Build history of the part. All positions in model axes, mm. A direction names the side the tool comes from. Give positions to 0.01 mm unless a question says otherwise; leave off trailing zeros. Order: outer loops, then holes, each group sorted by start corner. A loop starts at its lowest first (then second) coordinate and runs counter-clockwise, first axis right, second up. Notation, with made-up numbers: (89.5, 35.25) -> (95.5, 35.25) arc R26 cw to (95.5, 68.25) -> close; hole circle Ø5 at (55, 26.25). An arc over 180 degrees is marked (long way). Use a Markdown table: item, result. Add a question column.
```python
from build123d import *

# Parameters (mm, degrees)
SKETCH1_R           = 1.1
BOSS_EXTRUDE1_DEPTH = 5
SKETCH2_W           = 16
SKETCH2_H           = 12
BOSS_EXTRUDE2_DEPTH = 15
CUT_EXTRUDE1_START  = -5.5
SKETCH3_W           = 9
SKETCH3_H           = 14
CUT_EXTRUDE1_DEPTH  = 9.5
SKETCH4_R           = 1
CUT_EXTRUDE2_DEPTH  = 16
FILLET2_R           = 0.5
SKETCH5_R           = 1.9
CUT_EXTRUDE3_DEPTH  = 1
FILLET3_R           = 1
CUT_EXTRUDE4_START  = -0.5
SKETCH6_R           = 2
CUT_EXTRUDE4_DEPTH  = 5.5
FILLET4_R           = 0.5


with BuildPart() as part:
    # Sketch1 → Boss-Extrude1 (new body)
    with BuildSketch(Plane.XY):
        with BuildLine():
            ThreePointArc((0, 4.5), (-4.5, 0), (0, -4.5))
            Line((0, -4.5), (50, -4.5))
            Line((50, -4.5), (50, 4.5))
            Line((50, 4.5), (0, 4.5))
        make_face()
        Circle(SKETCH1_R, mode=Mode.SUBTRACT)
    extrude(amount=BOSS_EXTRUDE1_DEPTH)

    # Sketch2 → Boss-Extrude2 (add)
    with BuildSketch(Plane(origin=(0, 4.5, 0), x_dir=(1, 0, 0), z_dir=(0, 1, 0))):
        with Locations((58, 1)):
            Rectangle(SKETCH2_W, SKETCH2_H)
    extrude(amount=-BOSS_EXTRUDE2_DEPTH)

    # Sketch3 → Cut-Extrude1 (cut)
    with BuildSketch(Plane(origin=(0, 4.5, 0), x_dir=(1, 0, 0), z_dir=(0, 1, 0)).offset(CUT_EXTRUDE1_START)):
        with Locations((57.5, 2)):
            Rectangle(SKETCH3_W, SKETCH3_H)
    extrude(amount=-CUT_EXTRUDE1_DEPTH, mode=Mode.SUBTRACT)

    # Sketch4 → Cut-Extrude2 (cut)
    with BuildSketch(Plane(origin=(66, 0, 0), x_dir=(0, 0, -1), z_dir=(1, 0, 0))):
        with Locations((1, -6.5)):
            Circle(SKETCH4_R)
    extrude(amount=-CUT_EXTRUDE2_DEPTH, mode=Mode.SUBTRACT)

    # Fillet2
    fillet2_edges = [part.edges().sort_by_distance(p)[0] for p in [
        (53, -6.5, 0),
    ]]
    fillet(fillet2_edges, radius=FILLET2_R)

    # Sketch5 → Cut-Extrude3 (cut)
    with BuildSketch(Plane(origin=(66, 0, 0), x_dir=(0, 0, -1), z_dir=(1, 0, 0))):
        with Locations((1, -6.5)):
            Circle(SKETCH5_R)
    extrude(amount=-CUT_EXTRUDE3_DEPTH, mode=Mode.SUBTRACT)

    # Fillet3
    fillet3_edges = [part.edges().sort_by_distance(p)[0] for p in [
        (53, -10.5, -1),
        (51.5, -10.5, 5),
        (53, -5.75, 5),
        (53, -5.75, -7),
        (51.5, -10.5, -7),
        (64, -10.5, 5),
        (62, -5.75, -7),
        (62, -5.75, 5),
        (64, -10.5, -7),
        (62, -10.5, -1),
    ]]
    fillet(fillet3_edges, radius=FILLET3_R)

    # Sketch6 → Cut-Extrude4 (cut)
    with BuildSketch(Plane.ZY.offset(-50).offset(CUT_EXTRUDE4_START)):
        with Locations((-1, -6.5)):
            Circle(SKETCH6_R)
    extrude(amount=CUT_EXTRUDE4_DEPTH, mode=Mode.SUBTRACT)

    # Fillet4
    fillet4_edges = [part.edges().sort_by_distance(p)[0] for p in [
        (-1.1, 0, 5),
        (-1.1, 0, 0),
    ]]
    fillet(fillet4_edges, radius=FILLET4_R)


solid = part.part
```
(1) Band-saw the part on B-B on z = -1. Give the cut face in (x, y).
(2) Pin check, flat tips, straight feed: pin 1 Ø4.5 at (y, z) = (-5.5, -1.5) entering from -X; pin 2 Ø2.5 at (y, z) = (-6.5, -1) entering from -X; pin 3 Ø3.5 at (x, y) = (0, 0) entering from -Z; pin 4 Ø3 at (x, y) = (34, -6.5) entering from -Z. Stop position of each tip, or through.
(3) Wall check: probe 1 along X at (y, z) = (-3.5, -5); probe 2 along Y at (x, z) = (51.45, -1); probe 3 along Z at (x, y) = (50.35, -6.5). Give the ranges that are in metal, low to high.
(4) Band-saw the part on A-A on y = -6.5. State how many separate pieces and enclosed holes the cut face has, plus the area to 3 significant figures.
(5) Tool access for faces 1 (the face through (65.507, -4.616, -0.753)), 2 (the face through (62, -5, -1)), 3 (the face through (50.254, -8.452, -1.434)), 4 (the face through (25, -4.5, 2)), 5 (the face through (51, -10.5, -1)): list every direction of +Z, -Z, +X, -X, +Y, -Y with a clear straight run to the whole face (end or side of a thin tool).
(6) Band-saw the part on C-C on y = 0. Give the cut face in (x, z).
(7) Mould opens along Y. For faces 6 (the face through (57, -1, -1)), 7 (the face through (63.52, -5.51, -0.87)), 8 (the face through (22, 0, 0)) say: released by +Y, released by -Y, zero draft, split by the parting line, or undercut.
(8) Band-saw the part on D-D on z = -4. Give the cut face in (x, y), plus the area to 3 significant figures.
Response:
| question | item | result |
|---|---|---|
| 1 | outline | (50, -10.5) -> (52, -10.5) arc R1 ccw to (53, -9.5) -> (53, -8) arc R0.5 ccw to (52.5, -7.5) -> (50.5, -7.5) -> (50.5, -8.5) -> (50, -8.5) -> close; (50, -4.5) -> (50.5, -4.5) -> (50.5, -5.5) -> (52.5, -5.5) arc R0.5 ccw to (53, -5) -> (53, -1) -> (62, -1) -> (62, -5.5) -> (65, -5.5) -> (65, -4.6) -> (66, -4.6) -> (66, 4.5) -> (50, 4.5) -> close; (62, -9.5) arc R1 ccw to (63, -10.5) -> (66, -10.5) -> (66, -8.4) -> (65, -8.4) -> (65, -7.5) -> (62, -7.5) -> close |
| 2 | pin 1 | stops at x = -2.37 |
| 2 | pin 2 | stops at x = 50.5 |
| 2 | pin 3 | stops at z = 0 |
| 2 | pin 4 | passes through |
| 3 | probe 1 | x = 50 to 53, 62 to 66 |
| 3 | probe 2 | y = -10.5 to -7.5, -5.5 to 4.5 |
| 3 | probe 3 | z = -7 to -3, 1 to 5 |
| 4 | separate pieces | 4 |
| 4 | enclosed holes | 0 |
| 4 | area | 66.2 mm² |
| 5 | face 1 | +X |
| 5 | face 2 | +Z, -Z, -Y |
| 5 | face 3 | -X |
| 5 | face 4 | +Z, -Z, -X, -Y |
| 5 | face 5 | +Z, -Z, +X, -X, -Y |
| 6 | outline | (-4.5, 0) -> (-1.6, 0) arc R0.5 ccw to (-1.1, 0.5) -> (-1.1, 4.5) arc R0.5 ccw to (-1.6, 5) -> (-4.5, 5) -> close; (1.1, 0.5) arc R0.5 ccw to (1.6, 0) -> (50, 0) -> (50, -7) -> (66, -7) -> (66, 5) -> (1.6, 5) arc R0.5 ccw to (1.1, 4.5) -> close |
| 7 | face 6 | released by -Y |
| 7 | face 7 | undercut |
| 7 | face 8 | zero draft |
| 8 | outline | (50, -10.5) -> (52, -10.5) arc R1 ccw to (53, -9.5) -> (53, -1) -> (62, -1) -> (62, -9.5) arc R1 ccw to (63, -10.5) -> (66, -10.5) -> (66, 4.5) -> (50, 4.5) -> close |
| 8 | area | 154 mm² |
